Read the model definition and answer for the solid it produces. Units are mm, in the model's axes. Face numbers are marked on the shaded views. Give positions to 0.01 mm unless a question says otherwise; leave off trailing zeros. Loops run counter-clockwise (first coordinate to the right, second up) from the corner with the lowest first, then second, coordinate; pieces in that order, holes last. Notation, with made-up numbers: (-12.75, 48) - (-6.75, 48) arc R19 cw to (-6.75, 53) - close; hole circle Ø2 at (-14.75, 11). An arc over 180 degrees is marked (long way). Write item = value, one per line. Start each with the question number.
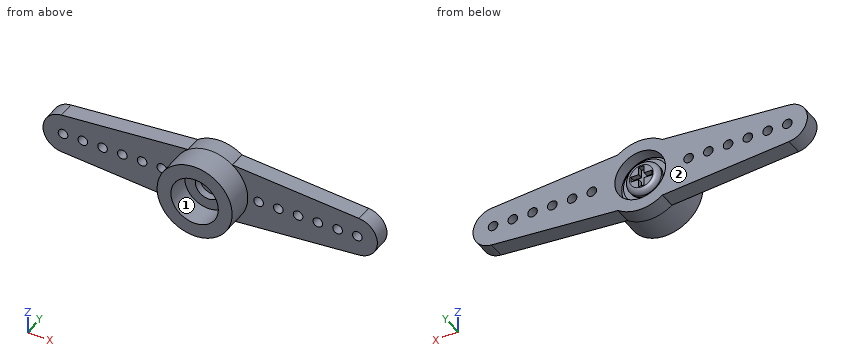
from build123d import *
from build123d.topology import SkipClean

# Parameters (mm, degrees)
EXTRUDE17_DEPTH = 1.6129
SKETCH19_R      = 3.6195
EXTRUDE19_DEPTH = 4.2291
SKETCH20_R      = 0.46355
SKETCH20_R_2    = 1.27
EXTRUDE20_DEPTH = 18.050548
SKETCH21_R      = 2.44475
EXTRUDE21_DEPTH = 1.1557
SKETCH22_R      = 2.286
EXTRUDE22_DEPTH = 2.3368
SKETCH23_R      = 2.159
EXTRUDE23_DEPTH = 0.2032
SKETCH24_R      = 1.651
EXTRUDE24_DEPTH = 0.762
EXTRUDE25_DEPTH = 0.508
FILLET1_R       = 0.508


with BuildPart() as part:
    # Sketch18 → Extrude17 (new body)
    with BuildSketch(Plane(origin=(0, 0, 0), x_dir=(1, 0, 0), z_dir=(0, 1, 0))):
        with BuildLine():
            Line((-14.34306, 1.923992), (-2.137414, 2.921))
            ThreePointArc((-2.137414, 2.921), (0, 3.6195), (2.137414, 2.921))
            Line((2.137414, 2.921), (14.34306, 1.923992))
            ThreePointArc((14.34306, 1.923992), (16.1163, 0), (14.34306, -1.923992))
            Line((14.34306, -1.923992), (2.137414, -2.921))
            ThreePointArc((2.137414, -2.921), (0, -3.6195), (-2.137414, -2.921))
            Line((-2.137414, -2.921), (-14.34306, -1.923992))
            ThreePointArc((-14.34306, -1.923992), (-16.1163, 0), (-14.34306, 1.923992))
        make_face()
    extrude(amount=EXTRUDE17_DEPTH)

    # Sketch19 → Extrude19 (add)
    with SkipClean():  # the faces are left unmerged after this step: merging them gives an invalid solid
        with BuildSketch(Plane(origin=(0, 1.6129, 0), x_dir=(1, 0, 0), z_dir=(0, 1, 0))):
            with Locations(Location((0, 0, 0), (0, 0, 53.805553))):
                Circle(SKETCH19_R)
        extrude(amount=-EXTRUDE19_DEPTH)

    # Sketch20 → Extrude20 (cut, through all)
    with SkipClean():  # the faces are left unmerged after this step: merging them gives an invalid solid
        with BuildSketch(Plane(origin=(0, 1.6129, 0), x_dir=(1, 0, 0), z_dir=(0, 1, 0))):
            with Locations(Location((-14.1859, 0, 0), (0, 0, 270))):
                Circle(SKETCH20_R)
            with Locations(Location((0, 0, 0), (0, 0, 270))):
                Circle(SKETCH20_R_2)
            with Locations(Location((12.2809, 0, 0), (0, 0, 270))):
                Circle(SKETCH20_R)
            with Locations(Location((-4.6609, 0, 0), (0, 0, 270))):
                Circle(SKETCH20_R)
            with Locations(Location((-6.5659, 0, 0), (0, 0, 270))):
                Circle(SKETCH20_R)
            with Locations(Location((-8.4709, 0, 0), (0, 0, 270))):
                Circle(SKETCH20_R)
            with Locations(Location((-10.3759, 0, 0), (0, 0, 270))):
                Circle(SKETCH20_R)
            with Locations(Location((-12.2809, 0, 0), (0, 0, 270))):
                Circle(SKETCH20_R)
            with Locations(Location((10.3759, 0, 0), (0, 0, 270))):
                Circle(SKETCH20_R)
            with Locations(Location((8.4709, 0, 0), (0, 0, 270))):
                Circle(SKETCH20_R)
            with Locations(Location((6.5659, 0, 0), (0, 0, 270))):
                Circle(SKETCH20_R)
            with Locations(Location((4.6609, 0, 0), (0, 0, 270))):
                Circle(SKETCH20_R)
            with Locations(Location((14.1859, 0, 0), (0, 0, 270))):
                Circle(SKETCH20_R)
        extrude(amount=-EXTRUDE20_DEPTH, mode=Mode.SUBTRACT)

    # Sketch21 → Extrude21 (cut)
    with SkipClean():  # the faces are left unmerged after this step: merging them gives an invalid solid
        with BuildSketch(Plane(origin=(0, 1.6129, 0), x_dir=(1, 0, 0), z_dir=(0, 1, 0))):
            with Locations(Location((0, 0, 0), (0, 0, 270))):
                Circle(SKETCH21_R)
        extrude(amount=-EXTRUDE21_DEPTH, mode=Mode.SUBTRACT)

    # Sketch22 → Extrude22 (cut)
    with SkipClean():  # the faces are left unmerged after this step: merging them gives an invalid solid
        with BuildSketch(Plane.XZ.offset(2.6162)):
            with Locations(Location((0, 0, 0), (0, 0, 270))):
                Circle(SKETCH22_R)
        extrude(amount=-EXTRUDE22_DEPTH, mode=Mode.SUBTRACT)



with BuildPart() as body_2:
    # Sketch23 → Extrude23 (new body)
    with BuildSketch(Plane(origin=(0, 0.4572, 0), x_dir=(1, 0, 0), z_dir=(0, 1, 0))):
        with Locations(Location((0, 0, 0), (0, 0, 270))):
            Circle(SKETCH23_R)
    extrude(amount=EXTRUDE23_DEPTH)


with BuildPart() as part_1:
    with SkipClean():  # the faces are left unmerged after this step: merging them gives an invalid solid
        add(part.part)

        add(body_2.part)  # Extrude24 merges body 2
        # Sketch24 → Extrude24 (add)
        with BuildSketch(Plane(origin=(0, 0.6604, 0), x_dir=(1, 0, 0), z_dir=(0, 1, 0))):
            with Locations(Location((0, 0, 0), (0, 0, 90))):
                Circle(SKETCH24_R)
        extrude(amount=EXTRUDE24_DEPTH)

    # Sketch25 → Extrude25 (cut)
    with SkipClean():  # the faces are left unmerged after this step: merging them gives an invalid solid
        with BuildSketch(Plane(origin=(0, 1.4224, 0), x_dir=(1, 0, 0), z_dir=(0, 1, 0))):
            Polygon((0.254, -1.016), (-0.254, -1.016), (-0.254, -0.254), (-1.016, -0.254), (-1.016, 0.254), (-0.254, 0.254), (-0.254, 1.016), (0.254, 1.016), (0.254, 0.254), (1.016, 0.254), (1.016, -0.254), (0.254, -0.254), align=None)
        extrude(amount=-EXTRUDE25_DEPTH, mode=Mode.SUBTRACT)

    # Fillet1
    fillet1_edges = [part_1.edges().sort_by_distance(p)[0] for p in [
        (0, 1.4224, 1.651),
    ]]
    fillet(fillet1_edges, radius=FILLET1_R)


solid = part_1.part
1. For a pull along X with two mould halves and no side action, classify the marked faces 1 and 2 as released by +X, released by -X, zero draft, split by the parting line, or undercut.
2. A cutting plane is placed at B-B on x = -3. Give the vertices of the cut face in (y, z).
3. A cutting plane is placed at A-A on y = -2.3. Give the vertices of the cut face in (x, z), and give its area (3 significant figures).
4. Given P1, Ø1, axis at x = -0.5, z = 0.5, coming from the +Y side; P2, Ø3, axis at x = 7.5, z = 2.5, coming from the -Y side; P3, Ø2, axis at x = 0.5, z = 0.5, coming from the -Y side, each flat-ended and moving along its own axis, determine where each tip first touches the part or whether it passes through.
5. Consider line 1 along X through (y, z) = (-0.4, -1.5); line 2 along Y through (x, z) = (7, -1.5); line 3 along Z through (x, y) = (-4.5, 1.05). Determine where each line is inside the solid, lowest interval first. Write a range as [from, to].
Reply:
q1.face_1 = undercut
q1.face_2 = zero draft
q2.outline = (-2.62, -2.03) - (0, -2.03) - (0, -2.85) - (1.61, -2.85) - (1.61, 2.85) - (0, 2.85) - (0, 2.03) - (-2.62, 2.03) - close
q3.outline = circle Ø7.24 at (0, 0); hole circle Ø4.57 at (0, 0)
q3.area = 24.7 mm^2
q4.P1 = 1.42
q4.P2 = 0
q4.P3 = -0.28
q5.line_1 = [-3.29, -1.73], [1.73, 3.29]
q5.line_2 = [0, 1.61]
q5.line_3 = [-2.73, -0.43], [0.43, 2.73]
